```python
from build123d import *

# Parameters (mm, degrees)
F0_R      = 32.5
F1_DEPTH  = 10
F2_R      = 29.5
F3_DEPTH  = 8
F4_R      = 4
F5_DEPTH  = 8
F7_D      = 3.5
F9_R      = 7.586322
F10_DEPTH = 25
F11_R     = 7.195806
F12_DEPTH = 8
F13_R     = 8.139218
F14_DEPTH = 8
F15_R     = 9.181934
F16_DEPTH = 8
F17_R     = 9.467051
F18_DEPTH = 8
F19_R     = 8.617722
F20_DEPTH = 8
F21_R     = 8.650571
F22_DEPTH = 8
F23_R     = 7.543209
F24_DEPTH = 2
F25_R     = 9.251874
F26_DEPTH = 2
F27_R     = 9.863577
F28_DEPTH = 2
F29_R     = 8.708559
F30_DEPTH = 25


with BuildPart() as f1:
    # F0 (on Top) → F1 (new body)
    with BuildSketch(Plane.XY):
        Circle(F0_R)
    extrude(amount=F1_DEPTH)

    # F2 (on face) → F3 (cut)
    with BuildSketch(Plane.XY.offset(10)):
        Circle(F2_R)
    extrude(amount=-F3_DEPTH, mode=Mode.SUBTRACT)

    # F4 (on face) → F5 (join)
    with BuildSketch(Plane.XY.offset(2)):
        Circle(F4_R)
    extrude(amount=F5_DEPTH)

    # F7 (through all)
    with Locations(Plane.XY.offset(10)):
        with Locations((0, 0)):
            Hole(F7_D / 2)

    # F9 (on Top) → F10 (cut)
    with BuildSketch(Plane.XY):
        with Locations((-17.948439, -5.982571)):
            Circle(F9_R)
    extrude(amount=-F10_DEPTH, mode=Mode.SUBTRACT)

    # F11 (on Top) → F12 (cut)
    with BuildSketch(Plane.XY):
        with Locations((-18.613562, 0)):
            Circle(F11_R)
    extrude(amount=F12_DEPTH, mode=Mode.SUBTRACT)

    # F13 (on face) → F14 (cut)
    with BuildSketch(Plane.XY.offset(2)):
        with Locations((0, 17.952453)):
            Circle(F13_R)
    extrude(amount=-F14_DEPTH, mode=Mode.SUBTRACT)

    # F15 (on Top) → F16 (cut)
    with BuildSketch(Plane.XY):
        with Locations((-3.715688, -14.254572)):
            Circle(F15_R)
    extrude(amount=-F16_DEPTH, mode=Mode.SUBTRACT)

    # F17 (on Top) → F18 (cut)
    with BuildSketch(Plane.XY):
        with Locations((0, -15.324812)):
            Circle(F17_R)
    extrude(amount=-F18_DEPTH, mode=Mode.SUBTRACT)

    # F19 (on Top) → F20 (cut)
    with BuildSketch(Plane.XY):
        with Locations((15.627168, 0)):
            Circle(F19_R)
    extrude(amount=-F20_DEPTH, mode=Mode.SUBTRACT)

    # F21 (on face) → F22 (cut)
    with BuildSketch(Plane.XY.offset(2)):
        with Locations((16.869104, 0)):
            Circle(F21_R)
    extrude(amount=-F22_DEPTH, mode=Mode.SUBTRACT)

    # F23 (on face) → F24 (join)
    with BuildSketch(Plane.XY.offset(2)):
        with Locations((-4.684343, -11.25865)):
            Circle(F23_R)
    extrude(amount=-F24_DEPTH)

    # F25 (on face) → F26 (join)
    with BuildSketch(Plane.XY.offset(2)):
        with Locations((0, -16.615551)):
            Circle(F25_R)
    extrude(amount=-F26_DEPTH)

    # F27 (on face) → F28 (join)
    with BuildSketch(Plane.XY.offset(2)):
        with Locations((-4.199367, -15.142487)):
            Circle(F27_R)
    extrude(amount=-F28_DEPTH)

    # F29 (on face) → F30 (cut)
    with BuildSketch(Plane.XY.offset(2)):
        with Locations((2.921705, -14.926143)):
            Circle(F29_R)
    extrude(amount=-F30_DEPTH, mode=Mode.SUBTRACT)


solid = f1.part
```
Model file for the job. Use its own axes, mm. A direction names the side the tool comes from. Round coordinates to 2 decimals unless told otherwise and drop trailing zeros. Order: outer loops, then holes, each group sorted by start corner. A loop starts at its lowest first (then second) coordinate and runs counter-clockwise, first axis right, second up. Notation, with made-up numbers: M 3.25,-8.5 L 32.25,-8.5 A18 ccw 32.25,12.5 Z; hole C 49.5,16 d9. An arc over 180 degrees is marked long. Use CSV: the item, a comma, the result in double quotes.
Item 1: Which spindle directions (+Z, -Z, +X, -X, +Y, -Y) get a long thin tool onto all of the face, cutting with end or side? Do faces 4 (the face through (28.14, 8.86, 6.06)), 5 (the face through (7, -29, 10)). Say none if no direction does.
Worked answers:
face 4,"+Z"
face 5,"+Z, +X, -X, +Y, -Y"
Item 2: Pull direction Y, two halves, no side cores. Call faces 1 (the face through (31, 9.76, 4.93)), 2 (the face through (2, -1, 10)), 3 (the face through (-1.06, 26.022, 1.014)): released by +Y, released by -Y, zero draft, split by the parting line, or undercut.
Worked answers:
face 1,"split by the parting line"
face 2,"zero draft"
face 3,"undercut"
Item 3: Saw through at D-D (x = 5.5). List the corners of the cut face in (y, z), plus the area to 3 significant figures.
Worked answers:
outline,"M -32.03,0 L -23.24,0 L -23.24,2 L -28.98,2 L -28.98,10 L -32.03,10 Z; M -6.61,0 L 11.95,0 L 11.95,2 L -6.61,2 Z; M 23.95,0 L 32.03,0 L 32.03,10 L 28.98,10 L 28.98,2 L 23.95,2 Z"
area,"120 mm²"
Item 4: Saw through at B-B (z = 4). List the corners of the cut face in (x, y).
Worked answers:
outline,"C 0,0 d65; C 0,0 d8; hole C 0,0 d59; hole C 0,0 d3.5"
Item 5: Probe probe 1 along Y at (x, z) = (0, 5); probe 2 along Y at (x, z) = (0, 1); probe 3 along X at (y, z) = (3, 6.5). List the from-to ranges inside material, lowest first.
Worked answers:
probe 1,"-32.5 to -29.5, -4 to -1.75, 1.75 to 4, 29.5 to 32.5"
probe 2,"-32.5 to -23.13, -6.72 to -1.75, 1.75 to 9.81, 26.09 to 32.5"
probe 3,"-32.36 to -29.35, -2.65 to 2.65, 29.35 to 32.36"
Item 6: Pin check, flat tips, straight feed: pin 1 (1.5 mm diameter, centred on x = 12, y = 7.5, fed in from +Z); pin 2 (1 mm diameter, centred on x = 9.5, z = 2, fed in from +Y); pin 3 (4 mm diameter, centred on y = -9, z = 5, fed in from +X); pin 4 (2 mm diameter, centred on x = 0, y = 0, fed in from -Z). Stop position of each tip, or through.
Worked answers:
pin 1,"z = 2"
pin 2,"y = 31.23"
pin 3,"x = 31.74"
pin 4,"through"
Item 7: Saw through at C-C (y = 21). List the corners of the cut face in (x, z), plus the area to 3 significant figures.
Worked answers:
outline,"M -24.8,0 L -7.55,0 L -7.55,2 L -20.72,2 L -20.72,10 L -24.8,10 Z; M 7.55,0 L 24.8,0 L 24.8,10 L 20.72,10 L 20.72,2 L 7.55,2 Z"
area,"134 mm²"
Item 8: Saw through at A-A (y = 0). List the corners of the cut face in (x, z), plus the area to 3 significant figures.
Worked answers:
outline,"M -32.5,0 L -25.81,0 L -25.81,2 L -29.5,2 L -29.5,10 L -32.5,10 Z; M -11.42,0 L -1.75,0 L -1.75,10 L -4,10 L -4,2 L -11.42,2 Z; M 1.75,0 L 8.22,0 L 8.22,2 L 4,2 L 4,10 L 1.75,10 Z; M 25.52,0 L 32.5,0 L 32.5,10 L 29.5,10 L 29.5,2 L 25.52,2 Z"
area,"144 mm²"
